Design review of the part built by this model. Coordinates are the model's own, in mm. Coordinates: 2 decimals unless noted, no trailing zeros. Order: outer loops, then holes, each group sorted by start corner. A loop starts at its lowest first (then second) coordinate and runs counter-clockwise, first axis right, second up. Notation, with made-up numbers: M 21.5,18 L 46.5,18 A16 cw 46.5,25 Z; hole C -9.75,30 d4. An arc over 180 degrees is marked long. Use CSV: the item, a comma, the result in double quotes.
```python
from build123d import *

# Parameters (mm, degrees)
F0_R     = 4.9657
F0_W     = 101.6
F0_H     = 82.55
F1_DEPTH = 3.175
F2_R     = 12.7


with BuildPart() as f1:
    # F0 (on Front) → F1 (new body, symmetric)
    with BuildSketch(Plane.XZ):
        Polygon((-82.55, 0), (0, 0), (0, 82.55), (-101.6, 82.55), (-101.6, 0), align=None)
        with BuildLine():
            ThreePointArc((-77.5843, 26.9875), (-79.0387198567, 23.4762198567), (-82.55, 22.0218))
            ThreePointArc((-82.55, 22.0218), (-87.5157, 26.9875), (-82.55, 31.9532))
            ThreePointArc((-82.55, 31.9532), (-79.0387198567, 30.4987801433), (-77.5843, 26.9875))
        make_face(mode=Mode.SUBTRACT)
        with Locations((-82.55, 69.85)):
            Circle(F0_R, mode=Mode.SUBTRACT)
        with Locations((50.8, 41.275)):
            Rectangle(F0_W, F0_H)
        with Locations((82.55, 26.9875)):
            Circle(F0_R, mode=Mode.SUBTRACT)
        with Locations((82.55, 69.85)):
            Circle(F0_R, mode=Mode.SUBTRACT)
    extrude(amount=F1_DEPTH, both=True)

    # F2
    f2_edges = [f1.edges().sort_by_distance(p)[0] for p in [
        (-101.6, 0, 82.55),
        (101.6, 0, 0),
        (101.6, 0, 82.55),
        (-101.6, 0, 0),
    ]]
    fillet(f2_edges, radius=F2_R)


solid = f1.part
```
(1) The part is to be moulded in two halves that separate along X. For faces 1 (the face through (101.6, 0, 41)), 2 (the face through (81.474, 0.044, 65.002)), 3 (the face through (1, 0, 82.55)), say which applies: pulls with the +X half, pulls with the -X half, needs draft (parallel to the pull), parting line crosses it, or undercut.
The answers:
face 1,"pulls with the +X half"
face 2,"undercut"
face 3,"needs draft"
(2) Wall thickness on probe 1 along Z at (x, y) = (82.55, 0.75); probe 2 along Z at (x, y) = (86.5, -0.25); probe 3 along X at (y, z) = (-0.25, 24.5): over which ranges is each line inside the solid? List them lowest first.
The answers:
probe 1,"z = 0 to 22.02, 31.95 to 64.88, 74.82 to 82.55"
probe 2,"z = 0 to 23.98, 30 to 66.84, 72.86 to 82.55"
probe 3,"x = -101.6 to -86.85, -78.25 to 78.25, 86.85 to 101.6"
(3) Add section A-A on y = 2. State the section outline as (x, z) points, and give its area (3 significant figures).
The answers:
outline,"M -101.6,12.7 A12.7 ccw -88.9,0 L 88.9,0 A12.7 ccw 101.6,12.7 L 101.6,69.85 A12.7 ccw 88.9,82.55 L -88.9,82.55 A12.7 ccw -101.6,69.85 Z; hole C -82.55,26.99 d9.93; hole C -82.55,69.85 d9.93; hole C 82.55,26.99 d9.93; hole C 82.55,69.85 d9.93"
area,"16,300 mm2"
(4) Clearance check with a flat-ended pin moving along its axis: P1, Ø3, axis at y = 0, z = 9.5, coming from the +X side. State where the tip first meets the part, or that it passes through.
The answers:
P1,"stops at x = 101.49"
(5) Add section B-B on z = 68. State the section outline as (x, y) points (3 decimals), and give its area (3 significant figures).
The answers:
outline,"M -101.6,-3.175 L -87.158,-3.175 L -87.158,3.175 L -101.6,3.175 Z; M -77.942,-3.175 L 77.942,-3.175 L 77.942,3.175 L -77.942,3.175 Z; M 87.158,-3.175 L 101.6,-3.175 L 101.6,3.175 L 87.158,3.175 Z"
area,"1,170 mm2"
(6) Add section C-C on x = 82.55. State the section outline as (y, z) points (3 decimals).
The answers:
outline,"M -3.175,0 L 3.175,0 L 3.175,22.022 L -3.175,22.022 Z; M -3.175,31.953 L 3.175,31.953 L 3.175,64.884 L -3.175,64.884 Z; M -3.175,74.816 L 3.175,74.816 L 3.175,82.55 L -3.175,82.55 Z"
